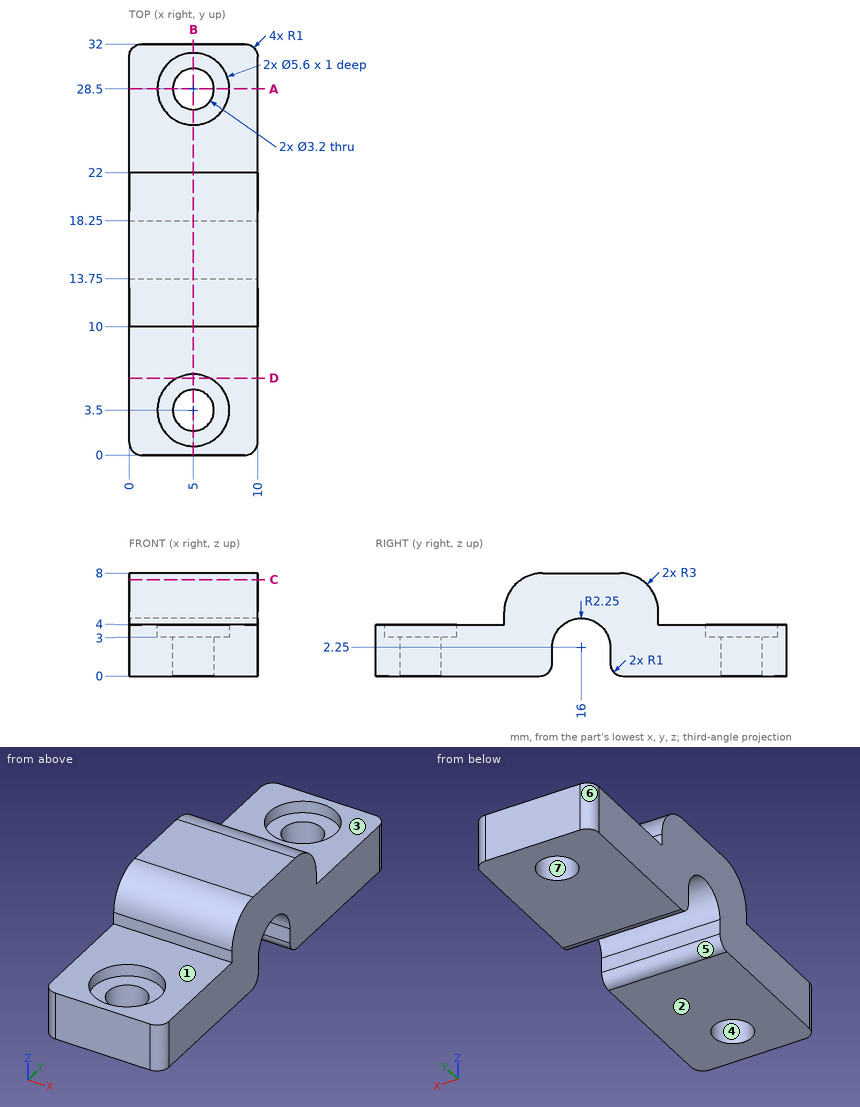
Verification items for this drawing (mm, ordinates from the low corner). A direction names the side the tool comes from. Coordinates: 2 decimals unless noted, no trailing zeros. Write each loop counter-clockwise with the first axis right and the second up, starting at its lowest first coordinate (ties: lowest second). Pieces come first, ordered by that corner, then holes. Notation, with made-up numbers: M 4.25,82.5 L 53.25,82.5 A33 ccw 53.25,119.5 Z; hole C 63.5,73.5 d5. An arc over 180 degrees is marked long. Answer as a JSON object with one key per item and string values. Group by question number.
(1) Cross-section at B-B, the plane x = 5. State how many separate pieces and enclosed holes the cut face has, and give its area (3 significant figures).
(2) Material ranges on line 1 (Y direction, x = 5, z = 1.45); line 2 (Y direction, x = 5, z = 3.5); line 3 (Z direction, x = 2, y = 16), recorded low to high.
(3) Tool access check on the marked faces 1, 2 and 3. Record the directions out of +Z, -Z, +X, -X, +Y, -Y that give a thin tool (end or side, any length) a straight path to the whole face; none if there is none.
(4) Gauge pin test, flat ends, axial feed: pin 1 (3 mm diameter, centred on x = 4, y = 4, fed in from +Z); pin 2 (1 mm diameter, centred on x = 4.5, z = 1.5, fed in from -Y); pin 3 (6 mm diameter, centred on x = 5.5, y = 30, fed in from +Z); pin 4 (0.8 mm diameter, centred on x = 5, z = 4.5, fed in from +Y). Record the tip position at first contact, or that the pin passes through.
(5) Cross-section at C-C, the plane z = 7.5. Record the cut outline in (x, y), and give its area (3 significant figures).
(6) Cross-section at D-D, the plane y = 6. Record the cut outline in (x, z), and give its area (3 significant figures).
(7) Release check for a two-part mould opening along X. For the marked faces 4, 5, 6 and 7 record: +X half, -X half, draft (parallel to the pull), parting line (faces both ways), or undercut.
(8) Cross-section at A-A, the plane y = 28.5. Record the cut outline in (x, z).
Reply:
{
 "1": {"separate pieces": "3", "enclosed holes": "0", "area": "123 mm²"},
 "2": {"line 1": "0 to 1.9, 5.1 to 13.75, 18.25 to 26.9, 30.1 to 32", "line 2": "0 to 0.7, 6.3 to 14.13, 17.87 to 25.7, 31.3 to 32", "line 3": "4.5 to 8"},
 "3": {"face 1": "+Z, +X, -X, -Y", "face 2": "-Z, +X, -X, +Y, -Y", "face 3": "+Z, +X, -X, +Y"},
 "4": {"pin 1": "z = 3", "pin 2": "y = 0", "pin 3": "z = 4", "pin 4": "y = 22"},
 "5": {"outline": "M 0,11.34 L 10,11.34 L 10,20.66 L 0,20.66 Z", "area": "93.2 mm²"},
 "6": {"outline": "M 0,0 L 10,0 L 10,4 L 6.26,4 L 6.26,3 L 3.74,3 L 3.74,4 L 0,4 Z", "area": "37.5 mm²"},
 "7": {"face 4": "undercut", "face 5": "draft", "face 6": "-X half", "face 7": "undercut"},
 "8": {"outline": "M 0,0 L 3.4,0 L 3.4,3 L 2.2,3 L 2.2,4 L 0,4 Z; M 6.6,0 L 10,0 L 10,4 L 7.8,4 L 7.8,3 L 6.6,3 Z"}
}
